from build123d import *

# Parameters (mm, degrees)
F0_W     = 101.6
F0_H     = 203.2
F1_DEPTH = 6.35
F2_W     = 76.2
F2_H     = 12.7
F2_W_2   = 67.544904
F2_H_2   = 5.582169
F2_W_3   = 68.530646
F2_H_3   = 6.063819
F3_DEPTH = 76.2


with BuildPart() as f1:
    # F0 (on Top) → F1 (new body)
    with BuildSketch(Plane.XY):
        with Locations((50.8, -101.6)):
            Rectangle(F0_W, F0_H)
    extrude(amount=F1_DEPTH)

    # F2 (on face) → F3 (join)
    with BuildSketch(Plane.XY.offset(6.35)):
        with Locations((63.5, -63.5)):
            Rectangle(F2_W, F2_H)
        with Locations((64.652548, -63.116084)):
            Rectangle(F2_W_2, F2_H_2, mode=Mode.SUBTRACT)
        with Locations((63.5, -139.7)):
            Rectangle(F2_W, F2_H)
        with Locations((64.159677, -139.843091)):
            Rectangle(F2_W_3, F2_H_3, mode=Mode.SUBTRACT)
    extrude(amount=F3_DEPTH)


solid = f1.part
Here's how the part is built. I have some questions about the finished solid (model axes, mm). A direction names the side the tool comes from. Coordinates: 2 decimals unless noted, no trailing zeros. Loops run counter-clockwise (first coordinate to the right, second up) from the corner with the lowest first, then second, coordinate; pieces in that order, holes last.
1. If we mould it in two halves opening along X, with no side actions, what happens to faces 5 (the flat face through (98.425, -63, 44)), 6 (the flat face through (50, -100, 0)), 7 (the flat face through (0, -103, 3))? For each: pulls with the +X half, pulls with the -X half, needs draft (parallel to the pull), parting line crosses it, or undercut.
2. For faces 1 (the flat face through (63, -69.85, 44)), 2 (the flat face through (64, -65.907, 44)), 3 (the flat face through (63, -146.05, 44)), 4 (the flat face through (25.4, -140, 44)), which set-ups out of +Z, -Z, +X, -X, +Y, -Y let a thin tool reach every point of the face, with its end or its side?
3. Imagine slicing it at D-D, the plane x = 20.5. Please give me the cut outline in (y, z).
4. Imagine slicing it at C-C, the plane y = -139.5. Please give me the cut outline in (x, z) (3 decimals).
5. Imagine slicing it at A-A, the plane z = 77.5. Please give me the cut outline in (x, y) (3 decimals).
6. For P1, Ø1.8, axis at y = -139.5, z = 43, coming from the -X side; P2, Ø12, axis at x = 59, z = 62, coming from the -Y side; P3, Ø4.5, axis at x = 69, y = -63.5, coming from the +Z side, each with a flat end and sliding along its axis, tell me the tip position at first contact or that it passes through.
7. Imagine slicing it at B-B, the plane x = 37.5. Please give me the cut outline in (y, z) (3 decimals).
8. I need wall thicknesses on L1, parallel to Y at x = 78, z = 32 (3 decimals); L2, parallel to X at y = -139, z = 66.5 (3 decimals); L3, parallel to Z at x = 24, y = -194. Which ranges of each line are inside material? Lowest first, please.
Taken from the geometry:
1. face 5: undercut
1. face 6: needs draft
1. face 7: pulls with the -X half
2. face 1: +Z, +X, -X
2. face 2: +Z
2. face 3: +Z, +X, -X, -Y
2. face 4: +Z, -X, +Y, -Y
3. outline: (-203.2, 0) - (0, 0) - (0, 6.35) - (-203.2, 6.35) - close
4. outline: (0, 0) - (101.6, 0) - (101.6, 82.55) - (98.425, 82.55) - (98.425, 6.35) - (29.894, 6.35) - (29.894, 82.55) - (25.4, 82.55) - (25.4, 6.35) - (0, 6.35) - close
5. outline: (25.4, -146.05) - (101.6, -146.05) - (101.6, -133.35) - (25.4, -133.35) - close; (25.4, -69.85) - (101.6, -69.85) - (101.6, -57.15) - (25.4, -57.15) - close; hole (29.894, -142.875) - (98.425, -142.875) - (98.425, -136.811) - (29.894, -136.811) - close; hole (30.88, -65.907) - (98.425, -65.907) - (98.425, -60.325) - (30.88, -60.325) - close
6. P1: stops at x = 25.4
6. P2: stops at y = -146.05
6. P3: stops at z = 6.35
7. outline: (-203.2, 0) - (0, 0) - (0, 6.35) - (-57.15, 6.35) - (-57.15, 82.55) - (-60.325, 82.55) - (-60.325, 6.35) - (-65.907, 6.35) - (-65.907, 82.55) - (-69.85, 82.55) - (-69.85, 6.35) - (-133.35, 6.35) - (-133.35, 82.55) - (-136.811, 82.55) - (-136.811, 6.35) - (-142.875, 6.35) - (-142.875, 82.55) - (-146.05, 82.55) - (-146.05, 6.35) - (-203.2, 6.35) - close
8. L1: y = -146.05 to -142.875, -136.811 to -133.35, -69.85 to -65.907, -60.325 to -57.15
8. L2: x = 25.4 to 29.894, 98.425 to 101.6
8. L3: z = 0 to 6.35
